Autodesk Inventor part; units mm, degrees
ref_plane "YZ Plane" through (0, 0, 0) normal (1, 0, 0) x (0, 1, 0)
ref_plane "XZ Plane" through (0, 0, 0) normal (0, 1, 0) x (-1, 0, 0)
ref_plane "XY Plane" through (0, 0, 0) normal (0, 0, 1) x (1, 0, 0)
sketch "スケッチ1" plane through (0, 0, 0) normal (0, 0, 1) x (1, 0, 0)
  line L0 (-20, 20) -> (20, 20)
  line L1 (20, 20) -> (20, -20)
  line L2 (20, -20) -> (-20, -20)
  line L3 (-20, -20) -> (-20, 20)
  line L4 (-20, 20) -> (20, -20) construction
  line L5 (20, 20) -> (-20, -20) construction
  line L6 (-18, 18) -> (18, 18)
  line L7 (18, 18) -> (18, -18)
  line L8 (18, -18) -> (-18, -18)
  line L9 (-18, -18) -> (-18, 18)
  line L10 (-18, 18) -> (18, -18) construction
  line L11 (18, 18) -> (-18, -18) construction
  point P0 (0, 0)
  point P1 (0, 0)
  dimension "d0" = 40
  dimension "d1" = 40
  dimension "d2" = 2
  dimension "d3" = 2
extrude "押し出し1" add sketch "スケッチ1" along normal blind 130
sketch "スケッチ3" plane through (-20, 20, 0) normal (0, 1, 0) x (1, 0, 0)
  line L0 (5, -115) -> (35, -115)
  line L1 (35, -115) -> (35, -15)
  line L2 (35, -15) -> (5, -15)
  line L3 (5, -15) -> (5, -115)
  line L4 (40, -130) -> (0, -130)
  line L5 (0, 0) -> (40, 0)
  line L6 (40, 0) -> (40, -130)
  line L7 (0, 0) -> (0, -130)
  point P0 (20, 0)
  dimension "d6" = 15
  dimension "d7" = 15
  dimension "d8" = 5
  dimension "d9" = 5
extrude "押し出し2" cut sketch "スケッチ3" against normal blind 100 contours L3 L2 L1 L0
fillet "フィレット1" radius 2 8 edges at (-15, 19, 115) (-15, 19, 15) (15, 19, 15) (15, 19, 115) (15, -19, 115) (-15, -19, 115) (-15, -19, 15) (15, -19, 15)
sketch "スケッチ4" plane through (-20, 20, 0) normal (0, 1, 0) x (1, 0, 0)
  line L0 (0, 0) -> (0, -130)
  line L1 (0, 0) -> (40, 0)
  line L2 (40, 0) -> (40, -130)
  line L3 (40, -130) -> (0, -130)
  point P0 (20, 0)
  point P1 (5, -5)
  point P2 (5, -125)
  point P3 (35, -125)
  point P4 (35, -5)
  dimension "d13" = 5
  dimension "d14" = 5
  dimension "d15" = 5
  dimension "d16" = 5
  dimension "d17" = 5
  dimension "d18" = 5
  dimension "d19" = 5
  dimension "d20" = 5
hole "穴1" at (-15, 20, 5) at (-15, 20, 125) at (15, 20, 125) at (15, 20, 5) direction (0, -1, 0) diameter 2.5 end up to surface
thread "ねじ1"
thread "ねじ2"
thread "ねじ3"
thread "ねじ4"
sketch "スケッチ5" plane through (20, -20, 0) normal (1, 0, 0) x (0, 0, -1)
  line L0 (0, 40) -> (0, 0)
  line L1 (0, 40) -> (-130, 40)
  line L2 (-130, 40) -> (-130, 0)
  point P0 (0, 20)
  point P1 (-65, 26)
  dimension "d37" = 14
  dimension "d67" = 65
hole "穴2" at (20, 6, 65) direction (-1, 0, 0) diameter 6 end through all
sketch "スケッチ6" plane through (-20, -20, 0) normal (-1, 0, 0) x (0, 0, 1)
  line L0 (0, 0) -> (0, 40)
  line L1 (0, 40) -> (130, 40)
  line L2 (130, 40) -> (130, 0)
  point P0 (0, 20)
  point P1 (112.5, 26)
  dimension "d46" = 14
  dimension "d54" = 17.5
hole "穴3" at (-20, 6, 112.5) direction (1, 0, 0) diameter 10 depth 8
sketch "スケッチ7" plane through (-20, -20, 0) normal (-1, 0, 0) x (0, 0, 1)
  line L0 (0, 40) -> (130, 40)
  line L1 (130, 40) -> (130, 0)
  point P0 (0, 20)
  point P1 (112.5, 19)
  dimension "d55" = 21
  dimension "d56" = 17.5
hole "穴4" at (-20, -1, 112.5) direction (1, 0, 0) diameter 3 depth 8
pattern_circular "円形状パターン1" count 3 over 360 about axis through (-16, 6, 112.5) along (-1, 0, 0) of "穴4"
sketch "スケッチ8" plane through (-20, -20, 0) normal (-1, 0, 0) x (0, 0, 1)
  line L0 (130, 40) -> (130, 0)
  line L1 (0, 0) -> (130, 0)
  line L2 (0, 40) -> (130, 40)
  point P0 (0, 20)
  point P1 (92.5, 26)
  dimension "d68" = 37.5
  dimension "d77" = 14
hole "穴5" at (-20, 6, 92.5) direction (1, 0, 0) diameter 6 end through all
properties part number "Gear box" material "アルミニウム"
Model file for the job. Use its own axes, mm. A direction names the side the tool comes from. Round coordinates to 2 decimals unless told otherwise and drop trailing zeros. Loops run counter-clockwise (first coordinate to the right, second up) from the corner with the lowest first, then second, coordinate; pieces in that order, holes last. Notation, with made-up numbers: (-34, -32.75) - (-25, -32.75) arc R16 ccw to (-25, -18.75) - close; hole circle Ø5 at (30, 53.5). An arc over 180 degrees is marked (long way). Write each question's results on one line, items separated by ' | '.
(1) Saw through at A-A, the plane y = -1. List the corners of the cut face in (x, z).
Answer below:
outline: (-20, 0) - (-18, 0) - (-18, 111) - (-20, 111) - close; (-20, 114) - (-18, 114) - (-18, 130) - (-20, 130) - close; (18, 0) - (20, 0) - (20, 130) - (18, 130) - close
(2) Saw through at B-B, the plane x = 6. List the corners of the cut face in (y, z), then the cut area to 3 significant figures.
Answer below:
outline: (-20, 0) - (-18, 0) - (-18, 15) - (-20, 15) - close; (-20, 115) - (-18, 115) - (-18, 130) - (-20, 130) - close; (18, 0) - (20, 0) - (20, 15) - (18, 15) - close; (18, 115) - (20, 115) - (20, 130) - (18, 130) - close | area: 120 mm^2
(3) 3-axis set-ups, long thin cutter, end or side, ignore diameter. For faces 5 (the cylindrical face through (-18.986, 7.915, 117.119)), 6 (the cylindrical face through (14.62, 18.99, 126.19)), 7 (the flat face through (-16, 18, 64)): which of +Z, -Z, +X, -X, +Y, -Y reach the whole face in a straight line?
Answer below:
face 5: -X | face 6: +Y | face 7: +Z, -Z
(4) Pin check, flat tips, straight feed: pin 1 (1.5 mm diameter, centred on x = 15, z = 5, fed in from +Y); pin 2 (10 mm diameter, centred on x = -9.5, z = 80, fed in from +Y); pin 3 (2.5 mm diameter, centred on y = -1, z = 112.5, fed in from -X). Stop position of each tip, or through.
Answer below:
pin 1: stops at y = -18 | pin 2: passes through | pin 3: stops at x = 18
(5) Wall check: L1, parallel to Z at x = -18.95, y = 6; L2, parallel to Y at x = -19.05, z = 112.5; L3, parallel to X at y = 17.5, z = 45. Give the ranges that are in metal, low to high.
Answer below:
L1: z = 0 to 62, 68 to 89.5, 95.5 to 107.5, 117.5 to 130 | L2: y = -20 to -2.5, 0.5 to 1, 11 to 20 | L3: x = -20 to -18, 18 to 20
(6) Saw through at D-D, the plane z = 5. List the corners of the cut face in (x, y), then the cut area to 3 significant figures.
Answer below:
outline: (-20, -20) - (20, -20) - (20, 20) - (16.25, 20) - (16.25, 18) - (18, 18) - (18, -18) - (-18, -18) - (-18, 18) - (-16.25, 18) - (-16.25, 20) - (-20, 20) - close; (-13.75, 18) - (13.75, 18) - (13.75, 20) - (-13.75, 20) - close | area: 294 mm^2
(7) Mould opens along X. For faces 1 (the flat face through (18, 0, 64)), 2 (the flat face through (16, -18, 64)), 3 (the flat face through (-2, -19, 0)), 4 (the flat face through (-20, 0, 64)) say: released by +X, released by -X, zero draft, split by the parting line, or undercut.
Answer below:
face 1: undercut | face 2: undercut | face 3: zero draft | face 4: released by -X
(8) Saw through at C-C, the plane y = 6. List the corners of the cut face in (x, z), then the cut area to 3 significant figures.
Answer below:
outline: (-20, 0) - (-18, 0) - (-18, 62) - (-20, 62) - close; (-20, 68) - (-18, 68) - (-18, 89.5) - (-20, 89.5) - close; (-20, 95.5) - (-18, 95.5) - (-18, 107.5) - (-20, 107.5) - close; (-20, 117.5) - (-18, 117.5) - (-18, 130) - (-20, 130) - close; (18, 0) - (20, 0) - (20, 62) - (18, 62) - close; (18, 68) - (20, 68) - (20, 89.5) - (18, 89.5) - close; (18, 95.5) - (20, 95.5) - (20, 130) - (18, 130) - close | area: 452 mm^2
